from build123d import *

# Parameters (mm, degrees)
SKETCH1_R           = 12.573
SKETCH1_R_2         = 10.31875
BOSS_EXTRUDE1_DEPTH = 26.9875
SKETCH2_R           = 17.526
SKETCH2_R_2         = 10.31875
BOSS_EXTRUDE2_DEPTH = 3.175
SKETCH3_R           = 17.526
SKETCH3_R_2         = 15
BOSS_EXTRUDE3_DEPTH = 6.477
CHAMFER1_SIZE       = 0.762
CHAMFER3_SIZE       = 0.254
CHAMFER4_SIZE       = 0.254
CHAMFER5_SIZE       = 1.397
CHAMFER6_SIZE       = 1.397


with BuildPart() as part:
    # Sketch1 → Boss-Extrude1 (new body)
    with BuildSketch(Plane(origin=(0, 0, 0), x_dir=(1, 0, 0), z_dir=(0, 1, 0))):
        Circle(SKETCH1_R)
        Circle(SKETCH1_R_2, mode=Mode.SUBTRACT)
    extrude(amount=BOSS_EXTRUDE1_DEPTH)

    # Sketch2 → Boss-Extrude2 (add)
    with BuildSketch(Plane(origin=(0, 26.9875, 0), x_dir=(1, 0, 0), z_dir=(0, 1, 0))):
        Circle(SKETCH2_R)
        Circle(SKETCH2_R_2, mode=Mode.SUBTRACT)
    extrude(amount=-BOSS_EXTRUDE2_DEPTH)

    # Sketch3 → Boss-Extrude3 (add)
    with BuildSketch(Plane(origin=(0, 26.9875, 0), x_dir=(1, 0, 0), z_dir=(0, 1, 0))):
        Circle(SKETCH3_R)
        Circle(SKETCH3_R_2, mode=Mode.SUBTRACT)
    extrude(amount=BOSS_EXTRUDE3_DEPTH)

    # Chamfer1
    chamfer1_edges = [part.edges().sort_by_distance(p)[0] for p in [
        (-17.526, 23.8125, 0),
        (-12.573, 0, 0),
    ]]
    chamfer(chamfer1_edges, length=CHAMFER1_SIZE)

    # Chamfer3
    chamfer3_edges = [part.edges().sort_by_distance(p)[0] for p in [
        (-17.526, 33.4645, 0),
    ]]
    chamfer(chamfer3_edges, length=CHAMFER3_SIZE)

    # Chamfer4
    chamfer4_edges = [part.edges().sort_by_distance(p)[0] for p in [
        (-15, 33.4645, 0),
    ]]
    chamfer(chamfer4_edges, length=CHAMFER4_SIZE)

    # Chamfer5
    chamfer5_edges = [part.edges().sort_by_distance(p)[0] for p in [
        (-15, 26.9875, 0),
    ]]
    chamfer(chamfer5_edges, length=CHAMFER5_SIZE)

    # Chamfer6
    chamfer6_edges = [part.edges().sort_by_distance(p)[0] for p in [
        (-10.31875, 26.9875, 0),
    ]]
    chamfer(chamfer6_edges, length=CHAMFER6_SIZE)


solid = part.part
Could you check a few things on this model? Use its own coordinates, in mm. A direction names the side the tool comes from. Give positions to 0.01 mm unless a question says otherwise; leave off trailing zeros. Order: outer loops, then holes, each group sorted by start corner. A loop starts at its lowest first (then second) coordinate and runs counter-clockwise, first axis right, second up. Notation, with made-up numbers: (-19, -25) - (17, -25) arc R28 ccw to (17, 12) - close; hole circle Ø7 at (39.25, 43.25). An arc over 180 degrees is marked (long way). One line per item, written item: value. Start each with the question number.
1. Thinking about a two-plate mould opening in Z: for faces 1 (the face through (-14.985, 30.764, -0.66)), 2 (the face through (-2.726, 12.126, 12.274)), 3 (the face through (-11.15, 26.988, -4.09)), 4 (the face through (0.82, 0, 10.44)), which applies, +Z half, -Z half, draft (parallel to the pull), parting line (faces both ways), or undercut?
2. If I drill on probe 1 along X at (y, z) = (29.4, 0); probe 2 along X at (y, z) = (13.75, 0), over which ranges is the centre line in solid material (lowest first)?
3. For faces 5 (the face through (2.4, 23.812, -12.5)), 6 (the face through (-2.237, 12.616, 10.073)), which set-ups out of +Z, -Z, +X, -X, +Y, -Y let a thin tool reach every point of the face, with its end or its side?
4. Imagine slicing it at C-C on y = 27.5. List the corners of the cut face in (x, z) for me.
5. Imagine slicing it at A-A on x = 0. List the corners of the cut face in (y, z) for me, plus the area to 3 significant figures.
6. Imagine slicing it at B-B on z = 0. List the corners of the cut face in (x, y) for me, plus the area to 3 significant figures.
7. For P1, Ø6, axis at y = 24.5, z = 2, coming from the +X side; P2, Ø8, axis at x = -2, z = 3, coming from the +Y side; P3, Ø1.5, axis at y = 10, z = -5, coming from the +X side; P4, Ø12, axis at y = 17, z = 11, coming from the -X side, each with a flat end and sliding along its axis, tell me the tip position at first contact or that it passes through.
Values:
1. face 1: undercut
1. face 2: parting line
1. face 3: undercut
1. face 4: draft
2. probe 1: -17.53 to -15, 15 to 17.53
2. probe 2: -12.57 to -10.32, 10.32 to 12.57
3. face 5: -Y
3. face 6: +Y, -Y
4. outline: circle Ø35.05 at (0, 0); hole circle Ø28.23 at (0, 0)
5. outline: (0, -11.81) - (0.76, -12.57) - (23.81, -12.57) - (23.81, -16.76) - (24.57, -17.53) - (33.21, -17.53) - (33.46, -17.27) - (33.46, -15.25) - (33.21, -15) - (28.38, -15) - (26.99, -13.6) - (26.99, -11.72) - (25.59, -10.32) - (0, -10.32) - close; (0, 10.32) - (25.59, 10.32) - (26.99, 11.72) - (26.99, 13.6) - (28.38, 15) - (33.21, 15) - (33.46, 15.25) - (33.46, 17.27) - (33.21, 17.53) - (24.57, 17.53) - (23.81, 16.76) - (23.81, 12.57) - (0.76, 12.57) - (0, 11.81) - close
5. area: 185 mm²
6. outline: (-17.53, 24.57) - (-16.76, 23.81) - (-12.57, 23.81) - (-12.57, 0.76) - (-11.81, 0) - (-10.32, 0) - (-10.32, 25.59) - (-11.72, 26.99) - (-13.6, 26.99) - (-15, 28.38) - (-15, 33.21) - (-15.25, 33.46) - (-17.27, 33.46) - (-17.53, 33.21) - close; (10.32, 0) - (11.81, 0) - (12.57, 0.76) - (12.57, 23.81) - (16.76, 23.81) - (17.53, 24.57) - (17.53, 33.21) - (17.27, 33.46) - (15.25, 33.46) - (15, 33.21) - (15, 28.38) - (13.6, 26.99) - (11.72, 26.99) - (10.32, 25.59) - close
6. area: 185 mm²
7. P1: x = 17.53
7. P2: through
7. P3: x = 11.83
7. P4: x = -11.54
